from build123d import *

# Parameters (mm, degrees)
CUT_EXTRUDE1_DEPTH      = 134.095432677
CIRPATTERN1_COUNT       = 2
CIRPATTERN1_ANGLE       = 90
CUT_EXTRUDE2_DEPTH      = 134.095432677
CUT_EXTRUDE2_DEPTH_BACK = 134.095432677
SKETCH4_W               = 71.692857504
SKETCH4_H               = 7.538034042
CHAMFER1_SIZE           = 1
CHAMFER2_SIZE           = 2


with BuildPart() as part:
    # Sketch2 → Revolve1 (revolve)
    with BuildSketch(Plane.XY, mode=Mode.PRIVATE) as revolve1_sk:
        with BuildLine():
            Line((0, 0), (-12.5, 0))
            Line((-12.5, 0), (-12.5, 100))
            ThreePointArc((-12.5, 100), (-26.960226668, 106.303549529), (-38.737016869, 116.798315107))
            Line((-38.737016869, 116.798315107), (-33.374125702, 121.298315107))
            ThreePointArc((-33.374125702, 121.298315107), (-18.481057884, 109.586391973), (0, 105.412291828))
            Line((0, 105.412291828), (0, 0))
        make_face()
    revolve(revolve1_sk.sketch.rotate(Axis((0, 0, 0), (0, 1, 0)), 270), axis=Axis((0, 0, 0), (0, 1, 0)))

    # Sketch3 → Cut-Extrude1 (cut, symmetric)
    with BuildSketch(Plane(origin=(0, 0, 0), x_dir=(0, 0, -1), z_dir=(1, 0, 0))):
        Polygon((-19, 121.298315107), (19, 121.298315107), (14.5, 116.798315107), (-14.5, 116.798315107), align=None)
    cut_extrude1 = extrude(amount=CUT_EXTRUDE1_DEPTH, both=True, mode=Mode.SUBTRACT)

    # CirPattern1: Cut-Extrude1 ×2 about axis
    cirpattern1_axis = Axis((0, 0, 0), (0, 1, 0))
    for i in range(1, CIRPATTERN1_COUNT):
        add(cut_extrude1.rotate(cirpattern1_axis, i * CIRPATTERN1_ANGLE / (CIRPATTERN1_COUNT - 1)), mode=Mode.SUBTRACT)

    # Sketch4 → Cut-Extrude2 (cut, two sides: drawn at the far end of the back side and taken through both)
    with BuildSketch(Plane(origin=(0, 0, 0), x_dir=(0, 0, -1), z_dir=(1, 0, 0)).offset(-CUT_EXTRUDE2_DEPTH_BACK)):
        with Locations((0, 123.067332128)):
            Rectangle(SKETCH4_W, SKETCH4_H)
    extrude(amount=CUT_EXTRUDE2_DEPTH + CUT_EXTRUDE2_DEPTH_BACK, mode=Mode.SUBTRACT)

    # Chamfer1
    # the kernel refuses this chamfer: 1, 0.710722016 mm, written as the material it takes off along each edge
    with BuildSketch(Plane(origin=(0, 116.798315107, 0), x_dir=(-0.900422371239431, 0, -0.43501672769166055), z_dir=(0.43501672769166055, 0, -0.900422371239431))) as chamfer1_piece_1_section:
        with BuildLine():
            Line((38.28405682, -0.547039951), (38.737016869 - CHAMFER1_SIZE, 0))
            Line((38.737016869 - CHAMFER1_SIZE, 0), (38.737016869, 0))
            ThreePointArc((38.737016869, 0), (38.510313841, -0.275766581), (38.28405682, -0.547039951))
        make_face()
    chamfer1_piece_1 = revolve(axis=Axis((0, 116.798315107, 0), (0, 1, 0)), revolution_arc=51.572716584, mode=Mode.PRIVATE)
    chamfer1_piece_1 = split(chamfer1_piece_1, bisect_by=Plane(origin=(0, 109.548315107, -7.25), z_dir=(0, 0.7071067811865445, 0.7071067811865507)), keep=Keep.TOP, mode=Mode.PRIVATE)
    chamfer1_piece_1 = split(chamfer1_piece_1, bisect_by=Plane(origin=(0, 109.548315107, 7.25), z_dir=(0, 0.7071067811865445, -0.7071067811865507)), keep=Keep.TOP, mode=Mode.PRIVATE)
    add(chamfer1_piece_1, mode=Mode.SUBTRACT)
    with BuildSketch(Plane(origin=(0, 116.798315107, 0), x_dir=(0.9004223712394364, 0, 0.4350167276916494), z_dir=(-0.4350167276916494, 0, 0.9004223712394364))) as chamfer1_piece_2_section:
        with BuildLine():
            Line((38.28405682, -0.547039951), (38.737016869 - CHAMFER1_SIZE, 0))
            Line((38.737016869 - CHAMFER1_SIZE, 0), (38.737016869, 0))
            ThreePointArc((38.737016869, 0), (38.510313841, -0.275766581), (38.28405682, -0.547039951))
        make_face()
    chamfer1_piece_2 = revolve(axis=Axis((0, 116.798315107, 0), (0, 1, 0)), revolution_arc=51.572716584, mode=Mode.PRIVATE)
    chamfer1_piece_2 = split(chamfer1_piece_2, bisect_by=Plane(origin=(0, 109.548315107, 7.25), z_dir=(0, 0.7071067811865445, -0.7071067811865507)), keep=Keep.TOP, mode=Mode.PRIVATE)
    chamfer1_piece_2 = split(chamfer1_piece_2, bisect_by=Plane(origin=(0, 109.548315107, -7.25), z_dir=(0, 0.7071067811865445, 0.7071067811865507)), keep=Keep.TOP, mode=Mode.PRIVATE)
    add(chamfer1_piece_2, mode=Mode.SUBTRACT)
    with BuildSketch(Plane(origin=(0, 116.798315107, 0), x_dir=(-0.43501672769166544, 0, 0.9004223712394286), z_dir=(-0.9004223712394286, 0, -0.43501672769166544))) as chamfer1_piece_3_section:
        with BuildLine():
            Line((38.28405682, -0.547039951), (38.737016869 - CHAMFER1_SIZE, 0))
            Line((38.737016869 - CHAMFER1_SIZE, 0), (38.737016869, 0))
            ThreePointArc((38.737016869, 0), (38.510313841, -0.275766581), (38.28405682, -0.547039951))
        make_face()
    chamfer1_piece_3 = revolve(axis=Axis((0, 116.798315107, 0), (0, 1, 0)), revolution_arc=51.572716584, mode=Mode.PRIVATE)
    chamfer1_piece_3 = split(chamfer1_piece_3, bisect_by=Plane(origin=(-7.25, 109.548315107, 0), z_dir=(0.7071067811865507, 0.7071067811865445, -2.5121479338940513e-15)), keep=Keep.TOP, mode=Mode.PRIVATE)
    chamfer1_piece_3 = split(chamfer1_piece_3, bisect_by=Plane(origin=(7.25, 109.548315107, 0), z_dir=(-0.7071067811865507, 0.7071067811865445, 2.5121479338940513e-15)), keep=Keep.TOP, mode=Mode.PRIVATE)
    add(chamfer1_piece_3, mode=Mode.SUBTRACT)
    with BuildSketch(Plane(origin=(0, 116.798315107, 0), x_dir=(0.4350124309167343, 0, -0.9004244471069814), z_dir=(0.9004244471069814, 0, 0.4350124309167343))) as chamfer1_piece_4_section:
        with BuildLine():
            Line((38.28405682, -0.547039951), (38.737016869 - CHAMFER1_SIZE, 0))
            Line((38.737016869 - CHAMFER1_SIZE, 0), (38.737016869, 0))
            ThreePointArc((38.737016869, 0), (38.510313841, -0.275766581), (38.28405682, -0.547039951))
        make_face()
    chamfer1_piece_4 = revolve(axis=Axis((0, 116.798315107, 0), (0, 1, 0)), revolution_arc=25.786084879, mode=Mode.PRIVATE)
    chamfer1_piece_4 = split(chamfer1_piece_4, bisect_by=Plane(origin=(7.25, 109.548315107, 0), z_dir=(-0.7071067811865507, 0.7071067811865445, 2.5121479338940513e-15)), keep=Keep.TOP, mode=Mode.PRIVATE)
    add(chamfer1_piece_4, mode=Mode.SUBTRACT)
    with BuildSketch(Plane(origin=(0, 116.798315107, 0), x_dir=(0, 0, -1), z_dir=(1, 0, 0))) as chamfer1_piece_5_section:
        with BuildLine():
            Line((38.28405682, -0.547039951), (38.737016869 - CHAMFER1_SIZE, 0))
            Line((38.737016869 - CHAMFER1_SIZE, 0), (38.737016869, 0))
            ThreePointArc((38.737016869, 0), (38.510313841, -0.275766581), (38.28405682, -0.547039951))
        make_face()
    chamfer1_piece_5 = revolve(axis=Axis((0, 116.798315107, 0), (0, 1, 0)), revolution_arc=25.786084879, mode=Mode.PRIVATE)
    chamfer1_piece_5 = split(chamfer1_piece_5, bisect_by=Plane(origin=(-7.25, 109.548315107, 0), z_dir=(0.7071067811865507, 0.7071067811865445, -2.5121479338940513e-15)), keep=Keep.TOP, mode=Mode.PRIVATE)
    add(chamfer1_piece_5, mode=Mode.SUBTRACT)

    # Chamfer2
    chamfer2_edges = [part.edges().sort_by_distance(p)[0] for p in [
        (0, 0, 12.5),
    ]]
    chamfer(chamfer2_edges, length=CHAMFER2_SIZE)


solid = part.part
CAD build for the part. Positions are in the model's coordinates, mm. A direction names the side the tool comes from. Round coordinates to 2 decimals unless told otherwise and drop trailing zeros. Order: outer loops, then holes, each group sorted by start corner. A loop starts at its lowest first (then second) coordinate and runs counter-clockwise, first axis right, second up. Notation, with made-up numbers: (21, 67.5) - (51, 67.5) arc R28 ccw to (51, 103.5) - close; hole circle Ø8 at (14.25, 79.5). An arc over 180 degrees is marked (long way). Return JSON: item names as keys, results as strings.
(1) Pin check, flat tips, straight feed: pin 1 Ø13.5 at (x, z) = (0, 32) entering from +Y; pin 2 Ø6 at (y, z) = (35, 14.5) entering from -X; pin 3 Ø2 at (x, y) = (2, 13.5) entering from -Z. Stop position of each tip, or through.
Answer key:
{"pin 1": "stops at y = 116.8", "pin 2": "stops at x = -4.9", "pin 3": "stops at z = -12.46"}
(2) Cut at B-B (y = 12). Give the cut face in (x, z), then the cut area to 3 significant figures.
Answer key:
{"outline": "circle Ø25 at (0, 0)", "area": "491 mm^2"}
(3) Cut at A-A (z = 0). Give the cut face in (x, y).
Answer key:
{"outline": "(-38.28, 116.25) arc R50 ccw to (-12.5, 100) - (-12.5, 2) - (-10.5, 0) - (10.5, 0) - (12.5, 2) - (12.5, 100) arc R50 ccw to (38.28, 116.25) - (37.74, 116.8) - (29.15, 116.8) arc R43 cw to (-29.15, 116.8) - (-37.74, 116.8) - close"}
(4) Pull direction X, two halves, no side cores. Call faces 4 (the face through (0, 116.798, -33)), 5 (the face through (-3.755, 51.686, -11.923)), 6 (the face through (30.5, 118.1, -15.8)): +X half, -X half, draft (parallel to the pull), parting line (faces both ways), or undercut.
Answer key:
{"face 4": "undercut", "face 5": "parting line", "face 6": "draft"}
(5) Tool access for faces 1 (the face through (24, 119.298, 24)), 2 (the face through (33, 116.798, 0)), 3 (the face through (0, 116.798, 33)): list every direction of +Z, -Z, +X, -X, +Y, -Y with a clear straight run to the whole face (end or side of a thin tool).
Answer key:
{"face 1": "+Z, -Z, +X, -X, +Y", "face 2": "+X, -X, +Y", "face 3": "+Z, -Z, +Y"}
(6) Wall check: probe 1 along X at (y, z) = (38, 0.5); probe 2 along Z at (x, y) = (-3, 34); probe 3 along Y at (x, z) = (16, 22.5). Give the ranges that are in metal, low to high. Write a range as from..to.
Answer key:
{"probe 1": "x = -12.49..12.49", "probe 2": "z = -12.13..12.13", "probe 3": "y = 106.73..115.45"}
